```python
from build123d import *

# Parameters (mm, degrees)
SKETCH2_R           = 3.175
BOSS_EXTRUDE1_DEPTH = 3.175


with BuildPart() as part:
    # Sketch2 → Boss-Extrude1 (new, symmetric)
    with BuildSketch(Plane(origin=(0, 0, 0), x_dir=(1, 0, 0), z_dir=(0, 1, 0))):
        with BuildLine():
            Line((-13.97, -25.4), (13.97, -25.4))
            ThreePointArc((13.97, -25.4), (17.562102448, -23.912102448), (19.05, -20.32))
            Line((19.05, -20.32), (19.05, 20.32))
            ThreePointArc((19.05, 20.32), (17.562102448, 23.912102448), (13.97, 25.4))
            Line((13.97, 25.4), (-13.97, 25.4))
            ThreePointArc((-13.97, 25.4), (-17.562102448, 23.912102448), (-19.05, 20.32))
            Line((-19.05, 20.32), (-19.05, -20.32))
            ThreePointArc((-19.05, -20.32), (-17.562102448, -23.912102448), (-13.97, -25.4))
        make_face()
        with Locations(Location((0, -19.05, 0), (0, 0, 270))):
            Circle(SKETCH2_R, mode=Mode.SUBTRACT)
    extrude(amount=BOSS_EXTRUDE1_DEPTH, both=True)


solid = part.part
```
Here's how the part is built. I have some questions about the finished solid (model axes, mm). Give positions to 0.01 mm unless a question says otherwise; leave off trailing zeros. Loops run counter-clockwise (first coordinate to the right, second up) from the corner with the lowest first, then second, coordinate; pieces in that order, holes last. Notation, with made-up numbers: M -24,-30.75 L 9,-30.75 A27 cw 9,7.25 Z; hole C 74,57 d8. An arc over 180 degrees is marked long. Use one line per item in the form item = value. Start each with the question number.
Q1. Will this pin go through, and if not, where does the flat tip stop? pin 1 Ø7.5 at (x, z) = (0, 19.05) entering from -Y (3 decimals).
Q2. I need wall thicknesses on line 1 along X through (y, z) = (-1.25, 19.05) (3 decimals); line 2 along X through (y, z) = (2, 20.5). Which ranges of each line are inside material? Lowest first, please.
Q3. If we section it at D-D (x = -16): Write out the boundary of the cut face in (y, z) (3 decimals).
Q4. If we section it at A-A (x = 0): Write out the boundary of the cut face in (y, z) (3 decimals), then the cut area to 3 significant figures.
Q5. If we section it at C-C (z = 19.05): Write out the boundary of the cut face in (x, y) (3 decimals).
Q6. Thinking about a two-plate mould opening in X: for faces 1 (the cylindrical face through (-17.522, 0.044, -23.951)), 2 (the cylindrical face through (17.601, 0.044, -23.872)), 3 (the cylindrical face through (0.14, -0.04, 15.88)), which applies, +X half, -X half, draft (parallel to the pull), parting line (faces both ways), or undercut?
Q7. If we section it at B-B (y = -2.5): Write out the boundary of the cut face in (x, z) (3 decimals).
Taken from the geometry:
q1.pin_1 = -3.175
q2.line_1 = -19.05 to -3.175, 3.175 to 19.05
q2.line_2 = -19.05 to -2.82, 2.82 to 19.05
q3.outline = M -3.175,-24.977 L 3.175,-24.977 L 3.175,24.977 L -3.175,24.977 Z
q4.outline = M -3.175,-25.4 L 3.175,-25.4 L 3.175,15.875 L -3.175,15.875 Z; M -3.175,22.225 L 3.175,22.225 L 3.175,25.4 L -3.175,25.4 Z
q4.area = 282 mm^2
q5.outline = M -19.05,-3.175 L -3.175,-3.175 L -3.175,3.175 L -19.05,3.175 Z; M 3.175,-3.175 L 19.05,-3.175 L 19.05,3.175 L 3.175,3.175 Z
q6.face_1 = -X half
q6.face_2 = +X half
q6.face_3 = undercut
q7.outline = M -19.05,-20.32 A5.08 ccw -13.97,-25.4 L 13.97,-25.4 A5.08 ccw 19.05,-20.32 L 19.05,20.32 A5.08 ccw 13.97,25.4 L -13.97,25.4 A5.08 ccw -19.05,20.32 Z; hole C 0,19.05 d6.35
